from build123d import *

# Parameters (mm, degrees)
SKETCH2_W           = 342.9
SKETCH2_H           = 342.9
BOSS_EXTRUDE2_DEPTH = 12.7
DRAFT2_ANGLE        = -45
CUT_EXTRUDE1_DEPTH  = 5.08
CUT_EXTRUDE2_DEPTH  = 243.799289538
CUT_EXTRUDE3_DEPTH  = 243.799289538


with BuildPart() as part:
    # Sketch2 → Boss-Extrude2 (new body)
    with BuildSketch(Plane.XY):
        Rectangle(SKETCH2_W, SKETCH2_H)
    extrude(amount=BOSS_EXTRUDE2_DEPTH)

    # Draft2
    draft2_faces = [part.faces().sort_by_distance(p)[0] for p in [
        (-171.45, 0, 6.35),
        (0, -171.45, 6.35),
        (171.45, 0, 6.35),
        (0, 171.45, 6.35),
    ]]
    draft(draft2_faces, Plane(origin=(0, 0, 0), x_dir=(-1, 0, 0), z_dir=(0, 0, -1)), DRAFT2_ANGLE)

    # Sketch3 → Cut-Extrude1 (cut)
    with BuildSketch(Plane.XY.offset(12.7)):
        with BuildLine():
            Line((-171.45, 7.650128352), (-22.188943137, -141.610928512))
            ThreePointArc((-22.188943137, -141.610928512), (-22.188943137, -151.13), (-31.708014625, -151.13))
            Line((-31.708014625, -151.13), (-171.45, -11.388014625))
            Line((-171.45, -11.388014625), (-171.45, 7.650128352))
        make_face()
        with BuildLine():
            Line((11.388014625, 171.45), (-7.650128352, 171.45))
            Line((-7.650128352, 171.45), (141.610928512, 22.188943137))
            ThreePointArc((141.610928512, 22.188943137), (151.13, 22.188943137), (151.13, 31.708014625))
            Line((151.13, 31.708014625), (11.388014625, 171.45))
        make_face()
    extrude(amount=-CUT_EXTRUDE1_DEPTH, mode=Mode.SUBTRACT)

    # Sketch4 → Cut-Extrude2 (cut, through all)
    with BuildSketch(Plane.XY.offset(12.7)):
        with BuildLine():
            Line((99.06, 171.45), (99.06, 100.881890785))
            ThreePointArc((99.06, 100.881890785), (99.562699567, 98.354649397), (100.994266817, 96.212157602))
            Line((100.994266817, 96.212157602), (134.693157602, 62.513266817))
            ThreePointArc((134.693157602, 62.513266817), (136.835649397, 61.081699567), (139.362890785, 60.579))
            Line((139.362890785, 60.579), (171.45, 60.579))
            Line((171.45, 60.579), (171.45, 171.45))
            Line((171.45, 171.45), (99.06, 171.45))
        make_face()
    extrude(amount=-CUT_EXTRUDE2_DEPTH, mode=Mode.SUBTRACT)

    # Sketch5 → Cut-Extrude3 (cut, through all)
    with BuildSketch(Plane(origin=(0, 0, 0), x_dir=(-1, 0, 0), z_dir=(0, 0, -1))):
        with BuildLine():
            Line((-154.340192074, -138.323477991), (-147.739346277, -12.371837087))
            ThreePointArc((-147.739346277, -12.371837087), (-140.887450687, -1.754086289), (-128.2628732, -2.30648873))
            ThreePointArc((-128.2628732, -2.30648873), (-58.298772875, -58.298772875), (-2.30648873, -128.2628732))
            ThreePointArc((-2.30648873, -128.2628732), (-1.754086289, -140.887450687), (-12.371837087, -147.739346277))
            Line((-12.371837087, -147.739346277), (-138.323477991, -154.340192074))
            ThreePointArc((-138.323477991, -154.340192074), (-149.897385309, -149.897385309), (-154.340192074, -138.323477991))
        make_face()
    extrude(amount=-CUT_EXTRUDE3_DEPTH, mode=Mode.SUBTRACT)


solid = part.part
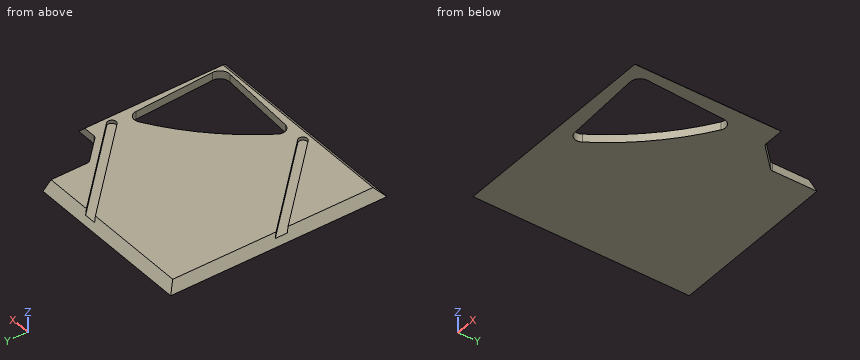
Geometry: final body of the model. Coordinates: model frame, mm. Give positions to 0.01 mm unless a question says otherwise; leave off trailing zeros. Loops run counter-clockwise (first coordinate to the right, second up) from the corner with the lowest first, then second, coordinate; pieces in that order, holes last. Notation, with made-up numbers: M -40,10.25 L -22,10.25 A18 cw -22,40.25 Z; hole C 77.5,-23 d9. An arc over 180 degrees is marked long. Put each result on its own line as item: value. Start each with the question number.
1) Ray query, line 1 along X through (y, z) = (-139, 9.5); line 2 along Y through (x, z) = (52, 9.5); line 3 along Y through (x, z) = (66, 9.5). Return the intervals inside material, ascending.
2) Cut plane A-A (z = 3.5). Output: boundary loops of the cut face in (x, y).
3) Cut plane C-C (x = 116.5). Output: boundary loops of the cut face in (y, z), then the cut area to 3 significant figures.
4) Cut plane D-D (y = 84). Output: boundary loops of the cut face in (x, z), then the cut area to 3 significant figures.
5) Cut plane B-B (y = -44). Output: boundary loops of the cut face in (x, z).
6) Contact query for flat-ended pins moving along their axis: pin 1 (3 mm diameter, centred on x = -40.5, z = 5.5, fed in from +Y); pin 2 (1.5 mm diameter, centred on x = 15.5, z = 11, fed in from +Y); pin 3 (6 mm diameter, centred on y = 101, z = 6, fed in from +X). Output: stop coordinate, or through.
Verdict:
1. line 1: -161.95 to -43.84, -24.8 to 0.96, 154.36 to 161.95
1. line 2: -161.95 to -149.82, -64.74 to 111.8, 130.84 to 161.95
1. line 3: -161.95 to -150.55, -50.8 to 97.8, 116.84 to 161.95
2. outline: M -167.95,-167.95 L 167.95,-167.95 L 167.95,60.58 L 139.36,60.58 A6.6 cw 134.69,62.51 L 100.99,96.21 A6.6 cw 99.06,100.88 L 99.06,167.95 L -167.95,167.95 Z; hole M 2.31,-128.26 A12.7 ccw 12.37,-147.74 L 138.32,-154.34 A15.24 ccw 154.34,-138.32 L 147.74,-12.37 A12.7 ccw 128.26,-2.31 A406.4 ccw Z
3. outline: M -171.45,0 L -153.2,0 L -153.2,12.7 L -158.75,12.7 Z; M -10.04,0 L 80.71,0 L 80.71,12.7 L 66.34,12.7 L 66.34,7.62 L 47.3,7.62 L 47.3,12.7 L -10.04,12.7 Z
3. area: 1,210 mm2
4. outline: M -171.45,0 L 113.21,0 L 113.21,12.7 L 98.84,12.7 L 98.84,7.62 L 79.8,7.62 L 79.8,12.7 L -158.75,12.7 Z
4. area: 3,440 mm2
5. outline: M -171.45,0 L 73.35,0 L 73.35,12.7 L -119.8,12.7 L -119.8,7.62 L -138.84,7.62 L -138.84,12.7 L -158.75,12.7 Z; M 149.4,0 L 171.45,0 L 158.75,12.7 L 149.4,12.7 Z
6. pin 1: y = 167.45
6. pin 2: y = 149.05
6. pin 3: x = 99.72
